The listing builds one solid part. Answer for the finished solid, in the listing's coordinates (mm). Face numbers are marked on the shaded views. A direction names the side the tool comes from. Round coordinates to 2 decimals unless told otherwise and drop trailing zeros. Write each loop counter-clockwise with the first axis right and the second up, starting at its lowest first coordinate (ties: lowest second). Pieces come first, ordered by that corner, then holes.
Item 1: A tool of negligible diameter and unlimited length cuts with its end or side. For the marked faces 1, 2 and 3, from which of +Z, -Z, +X, -X, +Y, -Y can it reach the whole face along a straight path? Write none if from no direction.
Item 2: Find the intervals of material crossed by probe 1 along Y at (x, z) = (41, 34.5); probe 2 along Z at (x, y) = (57, -43); probe 3 along X at (y, z) = (-35, 52), in increasing order.
Item 3: Find section B-B on y = -32.5. Give the vertices of the cut face in (x, z).
Item 4: Find section C-C on x = 28.5. Give the vertices of the cut face in (y, z).
Item 5: For a pull along Z with two mould halves and no side action, classify the marked faces 4, 5, 6 and 7 as +Z half, -Z half, draft (parallel to the pull), parting line (faces both ways), or undercut.
Item 6: Find section A-A on z = 42. Give the vertices of the cut face in (x, y), then the cut area to 3 significant figures.
Item 7: Each of these flat-tipped pins is pushed along its axis until it touches: pin 1 (12 mm diameter, centred on x = 8.5, y = -30.5, fed in from -Z); pin 2 (5 mm diameter, centred on y = -26, z = 31.5, fed in from -X). Where does it stop, or does it pass through?
Item 8: Find section D-D on y = -46. Give the vertices of the cut face in (x, z), then the cut area to 3 significant figures.
```python
from build123d import *

# Parameters (mm, degrees)
F1_DEPTH = 50.8
F3_DEPTH = 92.51427


with BuildPart() as f1:
    # F0 (on Front) → F1 (new body)
    with BuildSketch(Plane.XZ):
        Polygon((75.910531, 56.202993), (0, 56.202993), (0, 25.4), (-75.910531, 25.4), (-75.910531, 0), (75.910531, 0), align=None)
    extrude(amount=F1_DEPTH)

    # F2 (on Right) → F3 (cut)
    with BuildSketch(Plane.YZ):
        Polygon((-10.17795, 30.816574), (-10.17795, 49.853109), (-44.104453, 49.664631), (-44.104453, 30.816574), align=None)
    extrude(amount=F3_DEPTH, mode=Mode.SUBTRACT)


solid = f1.part
```
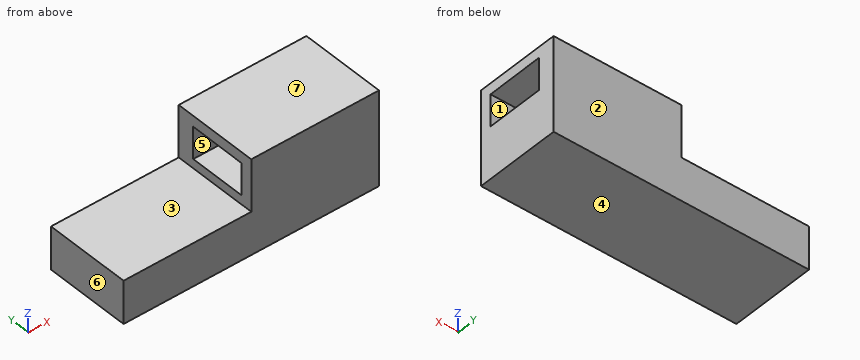
Check values:
1. face 1: +X, -X
1. face 2: +Z, -Z, +X, -X, +Y
1. face 3: +Z, -X, +Y, -Y
2. probe 1: y = -50.8 to -44.1, -10.18 to 0
2. probe 2: z = 0 to 30.82, 49.67 to 56.2
2. probe 3: x = 0 to 75.91
3. outline: (-75.91, 0) - (75.91, 0) - (75.91, 30.82) - (0, 30.82) - (0, 25.4) - (-75.91, 25.4) - close; (0, 49.73) - (75.91, 49.73) - (75.91, 56.2) - (0, 56.2) - close
4. outline: (-50.8, 0) - (0, 0) - (0, 56.2) - (-50.8, 56.2) - close; hole (-44.1, 30.82) - (-10.18, 30.82) - (-10.18, 49.85) - (-44.1, 49.66) - close
5. face 4: -Z half
5. face 5: undercut
5. face 6: draft
5. face 7: +Z half
6. outline: (0, -50.8) - (75.91, -50.8) - (75.91, -44.1) - (0, -44.1) - close; (0, -10.18) - (75.91, -10.18) - (75.91, 0) - (0, 0) - close
6. area: 1,280 mm2
7. pin 1: stops at z = 0
7. pin 2: stops at x = 0
8. outline: (-75.91, 0) - (75.91, 0) - (75.91, 56.2) - (0, 56.2) - (0, 25.4) - (-75.91, 25.4) - close
8. area: 6,190 mm2
